The listing builds one solid part. Answer for the finished solid, in the listing's coordinates (mm). A direction names the side the tool comes from. Round coordinates to 2 decimals unless told otherwise and drop trailing zeros. Write each loop counter-clockwise with the first axis right and the second up, starting at its lowest first coordinate (ties: lowest second). Pieces come first, ordered by that corner, then holes.
from build123d import *

# Parameters (mm, degrees)
PAD_DEPTH   = 25
FILLET_R    = 1.25
FILLET001_R = 1


with BuildPart() as part:
    # Sketch → Pad (new body)
    with BuildSketch(Plane.XZ):
        with BuildLine():
            Line((-75, 0), (0, 0))
            Line((0, 0), (8.242432, 0))
            Line((8.242432, 0), (0, 3))
            Line((0, 3), (-25.154795, 8.517473))
            ThreePointArc((-25.154795, 8.517473), (-37.643151, 9.988902), (-50.177682, 8.984088))
            ThreePointArc((-50.177682, 8.984088), (-50.984088, 7.822318), (-49.822318, 7.015912))
            ThreePointArc((-22.128287, 5.701128), (-35.900676, 7.930421), (-49.822318, 7.015912))
            Line((-22.128287, 5.701128), (-12.5, 3))
            Line((-12.5, 3), (-75, 3))
            Line((-75, 3), (-75, 0))
        make_face()
    extrude(amount=PAD_DEPTH)

    # Fillet
    fillet_edges = [part.edges().sort_by_distance(p)[0] for p in [
        (-75, -12.5, 3),
        (-75, -12.5, 0),
    ]]
    fillet(fillet_edges, radius=FILLET_R)

    # Fillet001
    fillet001_edges = [part.edges().sort_by_distance(p)[0] for p in [
        (-12.5, -12.5, 3),
        (8.242432, -12.5, 0),
    ]]
    fillet(fillet001_edges, radius=FILLET001_R)


solid = part.part
1. A tool of negligible diameter and unlimited length cuts with its end or side. For faces 4 (the face through (1.48, -12.32, 2.46)), 5 (the face through (-20.831, -12.325, 5.337)), from which of +Z, -Z, +X, -X, +Y, -Y can it reach the whole face along a straight path? Write none if from no direction.
Geometry says:
face 4: +Z, +X, +Y, -Y
face 5: -X, +Y, -Y
2. Section B-B on y = -18.5 is taken. Determine the outline of the cut face in (x, z), plus the area to 3 significant figures.
Geometry says:
outline: (-75, 1.25) arc R1.25 ccw to (-73.75, 0) - (2.57, 0) arc R1 ccw to (2.91, 1.94) - (0, 3) - (-25.15, 8.52) arc R63.85 ccw to (-50.18, 8.98) arc R1 ccw to (-49.82, 7.02) arc R61.85 cw to (-22.13, 5.7) - (-19.5, 4.96) arc R1 cw to (-19.77, 3) - (-73.75, 3) arc R1.25 ccw to (-75, 1.75) - close
area: 337 mm2
3. Given pin 1 (2 mm diameter, centred on x = -52.5, y = -13.5, fed in from +Z), flat-ended and moving along its own axis, determine where the tip first touches the part or whether it passes through.
Geometry says:
pin 1: stops at z = 3
4. Section C-C on x = -55 is taken. Determine the outline of the cut face in (y, z), plus the area to 3 significant figures.
Geometry says:
outline: (-25, 0) - (0, 0) - (0, 3) - (-25, 3) - close
area: 75.0 mm2
5. For a pull along X with two mould halves and no side action, classify faces 1 (the face through (-36.3, -25, 2.8)), 2 (the face through (-35.71, -12.32, 7.92)), 3 (the face through (-37.467, -12.325, 9.985)) as released by +X, released by -X, zero draft, split by the parting line, or undercut.
Geometry says:
face 1: zero draft
face 2: undercut
face 3: split by the parting line
6. Section A-A on x = -21 is taken. Determine the outline of the cut face in (y, z).
Geometry says:
outline: (-25, 0) - (0, 0) - (0, 3) - (-25, 3) - close; (-25, 5.38) - (0, 5.38) - (0, 7.61) - (-25, 7.61) - close
7. Straight lines are drawn through the part: line 1 along Z through (x, y) = (-51.5, -2); line 2 along Z through (x, y) = (-29.5, -21.5); line 3 along Z through (x, y) = (-23.5, -10.5). For each, find the intervals that lie inside material, in ascending order.
Geometry says:
line 1: z = 0 to 3
line 2: z = 0 to 3, 7.29 to 9.31
line 3: z = 0 to 3, 6.07 to 8.15
8. Section D-D on z = 4 is taken. Determine the outline of the cut face in (x, y), plus the area to 3 significant figures.
Geometry says:
outline: (-18.77, -25) - (-4.56, -25) - (-4.56, 0) - (-18.77, 0) - close
area: 355 mm2
